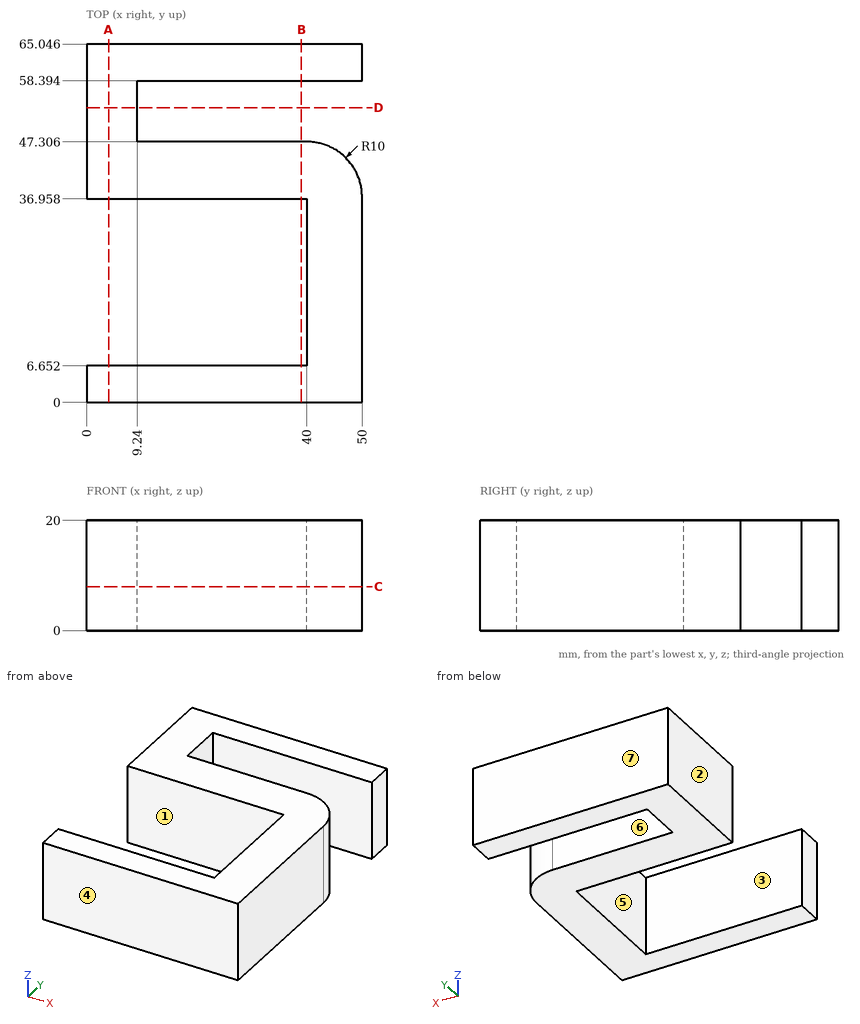
Input: dimensioned drawing with shaded views. Units: mm. Origin: part minimum x, y, z. A direction names the side the tool comes from. Give positions to 0.01 mm unless a question says otherwise; leave off trailing zeros. Order: outer loops, then holes, each group sorted by start corner. A loop starts at its lowest first (then second) coordinate and runs counter-clockwise, first axis right, second up.
(1) Section query B-B (x = 39). Return the cut outline in (y, z), plus the area to 3 significant figures.
(2) Material intervals for line 1 along Y through (x, z) = (23.5, 18.25); line 2 along Y through (x, z) = (8.5, 4.5); line 3 along X through (y, z) = (17.5, 8.75), sorted ascending.
(3) Section query C-C (z = 8). Return the cut outline in (x, y).
(4) Section query D-D (y = 53.5). Return the cut outline in (x, z), plus the area to 3 significant figures.
(5) Pull-direction query (Y, two-part tool) for the marked faces 1, 2, 3 and 4; classes: +Y half, -Y half, draft (parallel to the pull), parting line (faces both ways), or undercut.
(6) Contact query for flat-ended pins moving along their axis: P1, Ø10, axis at y = 47, z = 12.5, coming from the +X side; P2, Ø10, axis at y = 26.5, z = 12, coming from the -X side; P3, Ø3.5, axis at y = 53, z = 13.5, coming from the +X side. Output: stop coordinate, or through.
(7) Access query for the marked faces 5, 6 and 7. Directions: +Z, -Z, +X, -X, +Y, -Y. A direction counts if a zero-diameter tool reaches every point of the face in a straight line with its end or side. Return the directions, or none.
(8) Section query A-A (x = 4). Return the cut outline in (y, z).
Outcome:
1. outline: (0, 0) - (6.65, 0) - (6.65, 20) - (0, 20) - close; (36.96, 0) - (47.31, 0) - (47.31, 20) - (36.96, 20) - close; (58.39, 0) - (65.05, 0) - (65.05, 20) - (58.39, 20) - close
1. area: 473 mm2
2. line 1: y = 0 to 6.65, 36.96 to 47.31, 58.39 to 65.05
2. line 2: y = 0 to 6.65, 36.96 to 65.05
2. line 3: x = 40 to 50
3. outline: (0, 0) - (50, 0) - (50, 37.31) arc R10 ccw to (40, 47.31) - (9.24, 47.31) - (9.24, 58.39) - (50, 58.39) - (50, 65.05) - (0, 65.05) - (0, 36.96) - (40, 36.96) - (40, 6.65) - (0, 6.65) - close
4. outline: (0, 0) - (9.24, 0) - (9.24, 20) - (0, 20) - close
4. area: 185 mm2
5. face 1: undercut
5. face 2: draft
5. face 3: undercut
5. face 4: -Y half
6. P1: stops at x = 48.83
6. P2: stops at x = 40
6. P3: stops at x = 9.24
7. face 5: +Z, -Z, -X
7. face 6: +Z, -Z, +X
7. face 7: +Z, -Z, +X, -X, +Y
8. outline: (0, 0) - (6.65, 0) - (6.65, 20) - (0, 20) - close; (36.96, 0) - (65.05, 0) - (65.05, 20) - (36.96, 20) - close
